Source: CAD feature listing. Evaluate the final solid. Frame: model axes, mm. A direction names the side the tool comes from. Give positions to 0.01 mm unless a question says otherwise; leave off trailing zeros. Write each loop counter-clockwise with the first axis right and the second up, starting at its lowest first coordinate (ties: lowest second). Pieces come first, ordered by that corner, then holes. Notation, with made-up numbers: (-1.75, 55.5) -> (33.25, 55.5) arc R18 ccw to (33.25, 89.5) -> close; hole circle Ø1 at (36.5, 43). An arc over 180 degrees is marked (long way). Use one line per item in the form item = value. Start each with the question number.
(1) Draft query along Y for faces 6 (the face through (-29.29, 42.97, 85.12)), 7 (the face through (-30, 46, 4)), 8 (the face through (-34, 53, 2)), 9 (the face through (-29, 34.5, 47)). Return one class per face: pulls with the +Y half, pulls with the -Y half, needs draft (parallel to the pull), parting line crosses it, or undercut.
(2) First-contact query: P1, Ø4.5, axis at y = 48.5, z = 2.5, coming from the -X side; P2, Ø15, axis at x = -12.5, z = 48.5, coming from the +Y side; P3, Ø5, axis at y = 3, z = 65, coming from the +X side. Flat tips, straight axial feed; report the tip coordinate or a pass-through.
(3) Cut plane A-A, the plane x = 0. Output: boundary loops of the cut face in (y, z).
(4) Cut plane B-B, the plane z = 153. Output: boundary loops of the cut face in (x, y).
(5) Cut plane C-C, the plane x = -19.5. Output: boundary loops of the cut face in (y, z), and give its area (3 significant figures).
(6) Material intervals for line 1 along Y through (x, z) = (-33, 38); line 2 along Y through (x, z) = (-34, 0.95); line 3 along Z through (x, y) = (-14, 14.5), sorted ascending. Write a range as from..to.
(7) Cut plane D-D, the plane y = 36. Output: boundary loops of the cut face in (x, z).
(8) Set-up query: faces 1 (the face through (-23, 6.5, 65)), 2 (the face through (-38, 49, 2)), 3 (the face through (-31, -4, 65)), 4 (the face through (-12.762, 28.157, 1.972)), 5 (the face through (-36, 16.5, 162)). Return all of +Z, -Z, +X, -X, +Y, -Y with unobstructed straight access to the full face (end or side cutting, diameter ignored); none if empty.
from build123d import *

# Parameters (mm, degrees)
F0_R      = 1.75
F1_DEPTH  = 4
F3_DEPTH  = 160
F5_DEPTH  = 49
F7_DEPTH  = 19.001
F9_DEPTH  = 14.5
F11_DEPTH = 4
F13_DEPTH = 4


with BuildPart() as f1:
    # F0 (on Top) → F1 (new body)
    with BuildSketch(Plane.XY):
        Polygon((-38, -4), (4, -4), (4, 4), (-30, 53), (-38, 53), align=None)
        Circle(F0_R, mode=Mode.SUBTRACT)
        with Locations((-34, 49)):
            Circle(F0_R, mode=Mode.SUBTRACT)
    extrude(amount=F1_DEPTH)

    # F2 (on face) → F3 (join)
    with BuildSketch(Plane.XY.offset(4)):
        Polygon((-24.44898, 45), (-38, 45), (-38, -4), (-4, -4), (-4, 0), (-34, 0), (-34, 6.5), (-4, 6.5), (-4, 10.5), (-34, 10.5), (-34, 30.5), (-17.163265, 30.5), (-17.163265, 34.5), (-34, 34.5), (-34, 41), (-24.44898, 41), align=None)
    extrude(amount=F3_DEPTH)

    # F4 (on face) → F5 (join, through all)
    with BuildSketch(Plane.XZ.offset(4)):
        Polygon((-53, 0), (-38, 0), (-38, 164), align=None)
    extrude(amount=-F5_DEPTH)

    # F6 (on face) → F7 (cut, through all)
    with BuildSketch(Plane.YZ.offset(-34)):
        with BuildLine():
            Line((16.5, 164), (16.5, 160))
            ThreePointArc((16.5, 160), (20.5, 156), (24.5, 160))
            Line((24.5, 160), (24.5, 164))
            ThreePointArc((24.5, 164), (20.5, 168), (16.5, 164))
        make_face()
    extrude(amount=-F7_DEPTH, mode=Mode.SUBTRACT)

    # F8 (on face) → F9 (cut, through all)
    with BuildSketch(Plane.XZ.offset(4)):
        Polygon((-34, 164), (-4, 4), (-4, 164), align=None)
    extrude(amount=-F9_DEPTH, mode=Mode.SUBTRACT)

    # F10 (on face) → F11 (cut, through all)
    with BuildSketch(Plane.XZ.offset(-30.5)):
        Polygon((-17.163265, 164), (-34, 164), (-17.163265, 4), align=None)
    extrude(amount=-F11_DEPTH, mode=Mode.SUBTRACT)

    # F12 (on face) → F13 (cut, through all)
    with BuildSketch(Plane.XZ.offset(-41)):
        Polygon((-34, 164), (-24.44898, 4), (-24.44898, 164), align=None)
    extrude(amount=-F13_DEPTH, mode=Mode.SUBTRACT)


solid = f1.part
Geometry says:
q1.face_6 = needs draft
q1.face_7 = needs draft
q1.face_8 = pulls with the +Y half
q1.face_9 = undercut
q2.P1 = -38
q2.P2 = 10.5
q2.P3 = -34
q3.outline = (-4, 0) -> (-1.75, 0) -> (-1.75, 4) -> (-4, 4) -> close; (1.75, 0) -> (9.76, 0) -> (9.76, 4) -> (1.75, 4) -> close
q4.outline = (-39.01, -4) -> (-31.94, -4) -> (-31.94, 0) -> (-34, 0) -> (-34, 6.5) -> (-31.94, 6.5) -> (-31.94, 10.5) -> (-34, 10.5) -> (-34, 30.5) -> (-32.84, 30.5) -> (-32.84, 34.5) -> (-34, 34.5) -> (-34, 41) -> (-33.34, 41) -> (-33.34, 45) -> (-39.01, 45) -> close
q5.outline = (-4, 0) -> (37.87, 0) -> (37.87, 4) -> (34.5, 4) -> (34.5, 26.21) -> (30.5, 26.21) -> (30.5, 4) -> (10.5, 4) -> (10.5, 86.67) -> (6.5, 86.67) -> (6.5, 4) -> (0, 4) -> (0, 86.67) -> (-4, 86.67) -> close
q5.area = 918 mm^2
q6.line_1 = -4..0, 6.5..10.5, 30.5..34.5, 41..45
q6.line_2 = -4..47.25, 50.75..53
q6.line_3 = 0..4
q7.outline = (-53, 0) -> (-18.2, 0) -> (-18.2, 4) -> (-34, 4) -> (-34, 164) -> (-38, 164) -> close
q8.face_1 = +Z, +X
q8.face_2 = +Z, -Z, -X, +Y
q8.face_3 = +Z, -Z, +X, -X, -Y
q8.face_4 = +Z, -Z, +X, +Y
q8.face_5 = +Z, +X, -X
